Here's the drawing with two shaded views (mm, measured from the low corner). I have some questions. Coordinates: 2 decimals unless noted, no trailing zeros. Write each loop counter-clockwise with the first axis right and the second up, starting at its lowest first coordinate (ties: lowest second). Pieces come first, ordered by that corner, then holes.
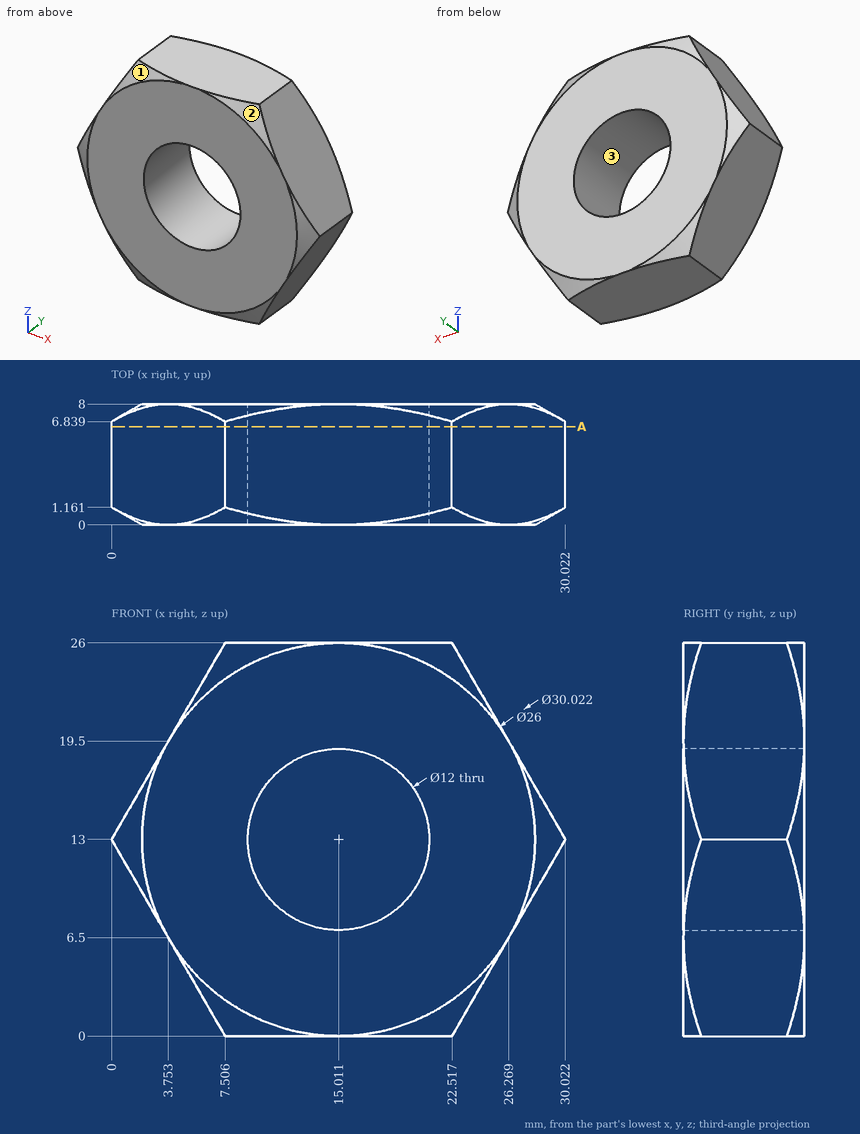
Item 1: I want a section at A-A, the plane y = 6.5. List the corners of the cut face in (x, z) for me (1 decimal), then the cut area to 3 significant figures.
Item 2: If I drill on line 1 along X through (y, z) = (2.25, 9.5) (1 decimal); line 2 along X through (y, z) = (4, 9) (1 decimal); line 3 along Z through (x, y) = (12, 6.5), over which ranges is the centre line in solid material (lowest first)?
Item 3: Will these pins go through, and if not, where does the flat tip stop? pin 1 Ø3 at (y, z) = (5.5, 9.5) entering from -X (1 decimal); pin 2 Ø9.5 at (x, z) = (15.01, 13) entering from -Y.
Item 4: If we mould it in two halves opening along X, with no side actions, what happens to the marked faces 1, 2 and 3? For each: released by +X, released by -X, zero draft, split by the parting line, or undercut.
Taken from the geometry:
1. outline: (0, 13) - (7.5, 0) - (22.5, 0) - (30, 13) - (22.5, 26) - (7.5, 26) - close; hole circle Ø12 at (15, 13)
1. area: 472 mm2
2. line 1: x = 2 to 10.1, 19.9 to 28
2. line 2: x = 2.3 to 10.5, 19.5 to 27.7
2. line 3: z = 0 to 7.81, 18.19 to 26
3. pin 1: stops at x = 1.2
3. pin 2: passes through
4. face 1: released by -X
4. face 2: released by +X
4. face 3: undercut
